Read the model definition and answer for the solid it produces. Units are mm, in the model's axes. A direction names the side the tool comes from. Round coordinates to 2 decimals unless told otherwise and drop trailing zeros. Order: outer loops, then holes, each group sorted by start corner. A loop starts at its lowest first (then second) coordinate and runs counter-clockwise, first axis right, second up.
from build123d import *

# Parameters (mm, degrees)
BOSS_EXTRUDE1_DEPTH = 23
SKETCH5_R           = 1.6
BOSS_EXTRUDE2_DEPTH = 1.5
CHAMFER1_SIZE       = 1.5


with BuildPart() as part:
    # Sketch1 → Boss-Extrude1 (new body)
    with BuildSketch(Plane.XY):
        with BuildLine():
            Line((-4.081066361, 56.693646837), (-1.434724284, 50.304811902))
            ThreePointArc((-1.434724284, 50.304811902), (-1.250569634, 50.080418812), (-0.972784517, 49.996153619))
            Line((-0.972784517, 49.996153619), (0.972784517, 49.996153619))
            ThreePointArc((0.972784517, 49.996153619), (1.250569634, 50.080418812), (1.434724284, 50.304811902))
            Line((1.434724284, 50.304811902), (4.081066361, 56.693646837))
            ThreePointArc((4.081066361, 56.693646837), (4.043474856, 57.149428628), (3.65087332, 57.383979681))
            ThreePointArc((3.65087332, 57.383979681), (0, 57.5), (-3.65087332, 57.383979681))
            ThreePointArc((-3.65087332, 57.383979681), (-4.043474856, 57.149428628), (-4.081066361, 56.693646837))
        make_face()
    extrude(amount=-BOSS_EXTRUDE1_DEPTH)

    # Sketch5 → Boss-Extrude2 (add)
    with BuildSketch(Plane(origin=(0, 0, -23), x_dir=(-1, 0, 0), z_dir=(0, 0, -1))):
        with BuildLine():
            Line((-28.307864731, 69.452608262), (-13, 32.496153619))
            Line((-13, 32.496153619), (13, 32.496153619))
            Line((13, 32.496153619), (28.307864731, 69.452608262))
            ThreePointArc((28.307864731, 69.452608262), (0, 75), (-28.307864731, 69.452608262))
        make_face()
        with Locations((-21.848934107, 66.925)):
            Circle(SKETCH5_R, mode=Mode.SUBTRACT)
        with Locations(Location((21.848934107, 66.925, 0), (0, 0, 180))):
            Circle(SKETCH5_R, mode=Mode.SUBTRACT)
        with Locations((-9.422527235, 36.925)):
            Circle(SKETCH5_R, mode=Mode.SUBTRACT)
        with Locations(Location((9.422527235, 36.925, 0), (0, 0, 180))):
            Circle(SKETCH5_R, mode=Mode.SUBTRACT)
    extrude(amount=BOSS_EXTRUDE2_DEPTH)

    # Chamfer1
    chamfer1_edges = [part.edges().sort_by_distance(p)[0] for p in [
        (23.448934107, 66.925, -23),
        (-23.448934107, 66.925, -23),
        (11.022527235, 36.925, -23),
        (-11.022527235, 36.925, -23),
    ]]
    chamfer(chamfer1_edges, length=CHAMFER1_SIZE - 0.0001)  # a hair under: the kernel refuses the full size


solid = part.part
Q1. Straight lines are drawn through the part: probe 1 along Z at (x, y) = (-24.5, 69); probe 2 along Y at (x, z) = (0, -5.5); probe 3 along Y at (x, z) = (-2.5, -5.25). For each, find the intervals that lie inside material, in ascending order.
Outcome:
probe 1: z = -24.5 to -23
probe 2: y = 50 to 57.5
probe 3: y = 52.88 to 57.45
Q2. For faces 1 (the face through (2.739, 53.455, -11.339)), 2 (the face through (-2.776, 53.544, -11.339)), 3 (the face through (0, 49.996, -11)), 4 (the face through (0.1, 57.5, -11.3)), 5 (the face through (20.76, 51.23, -23.74)), determine the directions among +Z, -Z, +X, -X, +Y, -Y from which every point of the face is accessible in a straight line to the end or side of a thin tool.
Outcome:
face 1: +Z, +X, -Y
face 2: +Z, -X, -Y
face 3: +Z, +X, -X, -Y
face 4: +Z, +Y
face 5: +Z, -Z, +X, -Y
Q3. A cutting plane is placed at A-A, the plane z = -11. Give the vertices of the cut face in (x, y).
Outcome:
outline: (-4.08, 56.69) - (-1.43, 50.3) arc R0.5 ccw to (-0.97, 50) - (0.97, 50) arc R0.5 ccw to (1.43, 50.3) - (4.08, 56.69) arc R0.5 ccw to (3.65, 57.38) arc R57.5 ccw to (-3.65, 57.38) arc R0.5 ccw to start
Q4. A cutting plane is placed at C-C, the plane x = 5.5. Give the vertices of the cut face in (y, z).
Outcome:
outline: (32.5, -24.5) - (74.8, -24.5) - (74.8, -23) - (32.5, -23) - close
Q5. A cutting plane is placed at D-D, the plane y = 47. Give the vertices of the cut face in (x, z), plus the area to 3 significant figures.
Outcome:
outline: (-19.01, -24.5) - (19.01, -24.5) - (19.01, -23) - (-19.01, -23) - close
area: 57.0 mm2
Q6. A cutting plane is placed at B-B, the plane y = 55.5. Give the vertices of the cut face in (x, z), plus the area to 3 significant figures.
Outcome:
outline: (-22.53, -24.5) - (22.53, -24.5) - (22.53, -23) - (3.59, -23) - (3.59, 0) - (-3.59, 0) - (-3.59, -23) - (-22.53, -23) - close
area: 233 mm2
Q7. Flat-ended cylindrical pins translate along their axes: pin 1 (1.9 mm diameter, centred on x = -9.42, y = 36.92, fed in from +Z); pin 2 (2 mm diameter, centred on x = 0.5, z = -6, fed in from -Y); pin 3 (6 mm diameter, centred on x = 18.5, y = 70.5, fed in from +Z); pin 4 (5 mm diameter, centred on x = 21.85, y = 66.92, fed in from +Z). Find the tip coordinate at first contact, or state that the pin passes through.
Outcome:
pin 1: passes through
pin 2: stops at y = 50
pin 3: stops at z = -23
pin 4: stops at z = -23.59
